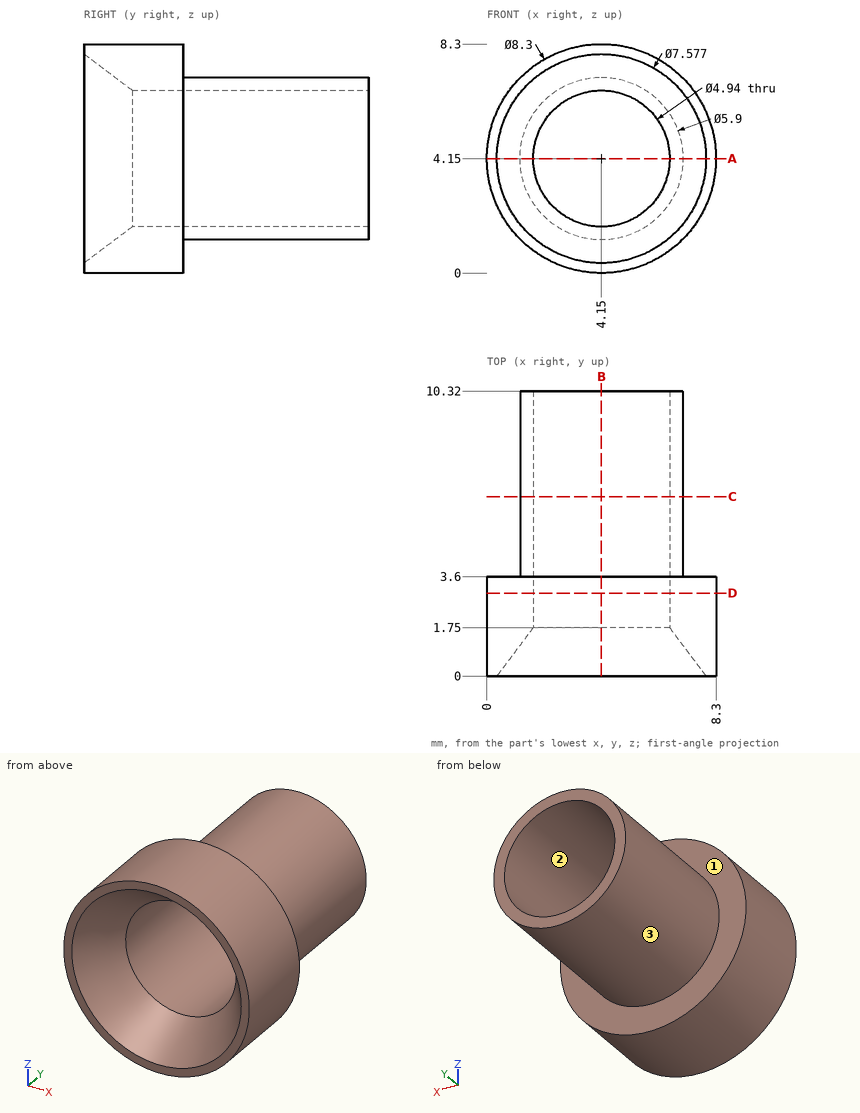
Source: three-view drawing plus pictorial views. Frame: mm from the lowest corner of the part. Give positions to 0.01 mm unless a question says otherwise; leave off trailing zeros. Order: outer loops, then holes, each group sorted by start corner. A loop starts at its lowest first (then second) coordinate and runs counter-clockwise, first axis right, second up. Notation, with made-up numbers: (13.5, 33) -> (70.5, 33) arc R10 cw to (70.5, 43) -> close; hole circle Ø5 at (-30.75, 62.25). An arc over 180 degrees is marked (long way). Use a Markdown table: item, result.
Q1. Section B-B (x = 4.15). Return the cut outline in (y, z).
A:
| item | result |
|---|---|
| outline | (0, 0) -> (3.6, 0) -> (3.6, 1.2) -> (10.32, 1.2) -> (10.32, 1.68) -> (1.75, 1.68) -> (0, 0.36) -> close; (0, 7.94) -> (1.75, 6.62) -> (10.32, 6.62) -> (10.32, 7.1) -> (3.6, 7.1) -> (3.6, 8.3) -> (0, 8.3) -> close |
Q2. First-contact query: P1, Ø3, axis at y = 7.5, z = 5, coming from the +X side; P2, Ø3, axis at x = 5, z = 3.5, coming from the -Y side. Flat tips, straight axial feed; report the tip coordinate or a pass-through.
A:
| item | result |
|---|---|
| P1 | x = 7.1 |
| P2 | y = 1.62 |
Q3. Material intervals for line 1 (X direction, y = 8.75, z = 4.15); line 2 (Y direction, x = 3.5, z = 8); line 3 (X direction, y = 9, z = 5.75), sorted ascending. Write a range as [from, to].
A:
| item | result |
|---|---|
| line 1 | [1.2, 1.68], [6.62, 7.1] |
| line 2 | [0, 3.6] |
| line 3 | [1.67, 2.27], [6.03, 6.63] |
Q4. Section A-A (z = 4.15). Return the cut outline in (x, y).
A:
| item | result |
|---|---|
| outline | (0, 0) -> (0.36, 0) -> (1.68, 1.75) -> (1.68, 10.32) -> (1.2, 10.32) -> (1.2, 3.6) -> (0, 3.6) -> close; (6.62, 1.75) -> (7.94, 0) -> (8.3, 0) -> (8.3, 3.6) -> (7.1, 3.6) -> (7.1, 10.32) -> (6.62, 10.32) -> close |
Q5. Pull-direction query (Z, two-part tool) for the marked faces 1, 2 and 3; classes: +Z half, -Z half, draft (parallel to the pull), parting line (faces both ways), or undercut.
A:
| item | result |
|---|---|
| face 1 | draft |
| face 2 | undercut |
| face 3 | parting line |
Q6. Section C-C (y = 6.5). Return the cut outline in (x, z).
A:
| item | result |
|---|---|
| outline | circle Ø5.9 at (4.15, 4.15); hole circle Ø4.94 at (4.15, 4.15) |
Q7. Section D-D (y = 3). Return the cut outline in (x, z).
A:
| item | result |
|---|---|
| outline | circle Ø8.3 at (4.15, 4.15); hole circle Ø4.94 at (4.15, 4.15) |
